```python
from build123d import *

# Parameters (mm, degrees)
SKETCH1_W                 = 50.18
SKETCH1_H                 = 60.2
BOSS_EXTRUDE1_DEPTH       = 55.3
SKETCH2_W                 = 38.18
SKETCH2_H                 = 55.3
CUT_EXTRUDE1_DEPTH        = 1.3
M8X1_0_TAPPED_HOLE1_D     = 7
M8X1_0_TAPPED_HOLE1_DEPTH = 10
M8X1_0_TAPPED_HOLE1_TIP   = 2.103012167


with BuildPart() as part:
    # Sketch1 → Boss-Extrude1 (new body)
    with BuildSketch(Plane.XY):
        with Locations((25.09, 30.1)):
            Rectangle(SKETCH1_W, SKETCH1_H)
    extrude(amount=BOSS_EXTRUDE1_DEPTH)

    # Sketch2 → Cut-Extrude1 (cut)
    with BuildSketch(Plane(origin=(0, 60.2, 0), x_dir=(1, 0, 0), z_dir=(0, 1, 0))):
        with Locations((25.09, -27.65)):
            Rectangle(SKETCH2_W, SKETCH2_H)
    extrude(amount=-CUT_EXTRUDE1_DEPTH, mode=Mode.SUBTRACT)

    # M8x1.0 Tapped Hole1
    with Locations(Plane.XY.offset(55.3)):
        with Locations((25.09, 30.2)):
            Hole(M8X1_0_TAPPED_HOLE1_D / 2, depth=M8X1_0_TAPPED_HOLE1_DEPTH)
            with Locations((0, 0, -(M8X1_0_TAPPED_HOLE1_DEPTH + M8X1_0_TAPPED_HOLE1_TIP / 2))):  # 118° drill point
                Cone(0, M8X1_0_TAPPED_HOLE1_D / 2, M8X1_0_TAPPED_HOLE1_TIP, mode=Mode.SUBTRACT)


solid = part.part
```
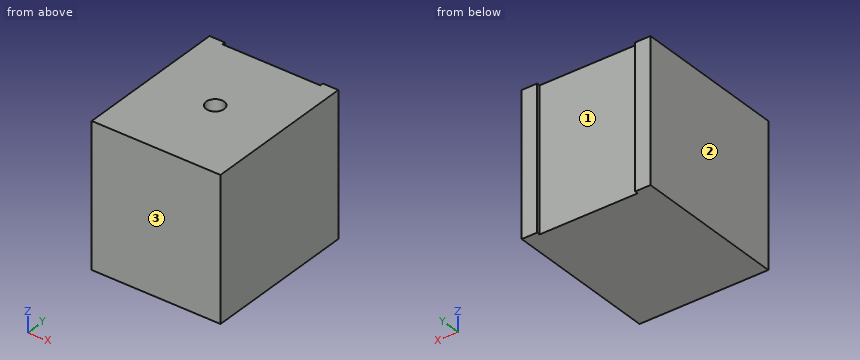
The listing builds one solid part. Answer for the finished solid, in the listing's coordinates (mm). Face numbers are marked on the shaded views. Give positions to 0.01 mm unless a question says otherwise; leave off trailing zeros. Order: outer loops, then holes, each group sorted by start corner. A loop starts at its lowest first (then second) coordinate and runs counter-clockwise, first axis right, second up.
Item 1: Find the intervals of material crossed by probe 1 along X at (y, z) = (30.2, 48); probe 2 along Y at (x, z) = (25.09, 49.5); probe 3 along Y at (x, z) = (33.5, 34.5), in increasing order.
From the geometry:
probe 1: x = 0 to 21.59, 28.59 to 50.18
probe 2: y = 0 to 26.7, 33.7 to 58.9
probe 3: y = 0 to 58.9
Item 2: For a pull along X with two mould halves and no side action, classify the marked faces 1, 2 and 3 as pulls with the +X half, pulls with the -X half, needs draft (parallel to the pull), parting line crosses it, or undercut.
From the geometry:
face 1: undercut
face 2: pulls with the -X half
face 3: needs draft
Item 3: The part is cut by section B-B, the plane x = 17.5. Give the vertices of the cut face in (y, z).
From the geometry:
outline: (0, 0) - (58.9, 0) - (58.9, 55.3) - (0, 55.3) - close
Item 4: Given pin 1 Ø11.5 at (x, z) = (20, 25) entering from +Y; pin 2 Ø1 at (y, z) = (59.5, 38) entering from -X; pin 3 Ø4 at (x, y) = (25.09, 30.2) entering from +Z, each flat-ended and moving along its own axis, determine where each tip first touches the part or whether it passes through.
From the geometry:
pin 1: stops at y = 58.9
pin 2: stops at x = 0
pin 3: stops at z = 44.4
Item 5: The part is cut by section A-A, the plane z = 38. Give the vertices of the cut face in (x, y), and give its area (3 significant figures).
From the geometry:
outline: (0, 0) - (50.18, 0) - (50.18, 60.2) - (44.18, 60.2) - (44.18, 58.9) - (6, 58.9) - (6, 60.2) - (0, 60.2) - close
area: 2,970 mm2
